Work out the finished part from the listing and answer in its coordinate system (mm). A direction names the side the tool comes from. Round coordinates to 2 decimals unless told otherwise and drop trailing zeros. Write each loop counter-clockwise with the first axis right and the second up, starting at its lowest first coordinate (ties: lowest second). Pieces come first, ordered by that corner, then holes. Notation, with made-up numbers: (-22.75, 49) -> (26.25, 49) arc R11 ccw to (26.25, 63) -> close; hole circle Ø3 at (72, -22). An arc over 180 degrees is marked (long way). Answer as a JSON object with one key per item and string values. Group by question number.
from build123d import *

# Parameters (mm, degrees)
SKETCH3_W               = 55.024039141
SKETCH3_H               = 32.210333873
BOSS_EXTRUDE1_DEPTH     = 1.5
SKETCH4_W               = 14
SKETCH4_H               = 14
CUT_EXTRUDE1_DEPTH      = 1.5
CUT_EXTRUDE4_DEPTH      = 327.051192929
CUT_EXTRUDE4_DEPTH_BACK = 327.051192929


with BuildPart() as part:
    # Sketch3 → Boss-Extrude1 (new body)
    with BuildSketch(Plane.XY):
        with Locations((282.811419242, 83.927296462)):
            Rectangle(SKETCH3_W, SKETCH3_H)
    extrude(amount=BOSS_EXTRUDE1_DEPTH)

    # Sketch4 → Cut-Extrude1 (cut)
    with BuildSketch(Plane.XY.offset(1.5)):
        with Locations((271.905830275, 82.45473243)):
            Rectangle(SKETCH4_W, SKETCH4_H)
        with Locations((290.956988381, 82.45473243)):
            Rectangle(SKETCH4_W, SKETCH4_H)
    extrude(amount=-CUT_EXTRUDE1_DEPTH, mode=Mode.SUBTRACT)

    # Sketch1 → Cut-Extrude4 (cut, two sides: drawn at the far end of the back side and taken through both)
    with BuildSketch(Plane.XY.offset(-CUT_EXTRUDE4_DEPTH_BACK)):
        Polygon((272.906316619, 84.755597823), (272.906316619, 87.985794184), (266.155906266, 87.985794184), (266.155906266, 84.755597823), (265.330856112, 84.755597823), (265.330856112, 81.955427603), (266.155906266, 81.955427603), (266.155906266, 75.684746413), (267.880011074, 75.684746413), (267.880011074, 74.484573455), (271.18021169, 74.484573455), (271.18021169, 75.684746413), (272.906316619, 75.684746413), (272.906316619, 80.155418181), (274.431409328, 80.155418181), (274.431409328, 75.45473243), (288.431409328, 75.45473243), (288.431409328, 80.155418181), (289.956502038, 80.155418181), (289.956502038, 75.684746413), (291.680606845, 75.684746413), (291.680606845, 74.484573455), (294.980807461, 74.484573455), (294.980807461, 75.684746413), (296.70691239, 75.684746413), (296.70691239, 81.955427603), (297.530962483, 81.955427603), (297.530962483, 84.755446764), (296.70691239, 84.755446764), (296.70691239, 87.985643125), (289.956502038, 87.985643125), (289.956502038, 84.755446764), (288.431409328, 84.755446764), (288.431409328, 89.45473243), (274.431409328, 89.45473243), (274.431409328, 84.755597823), align=None)
    extrude(amount=CUT_EXTRUDE4_DEPTH + CUT_EXTRUDE4_DEPTH_BACK, mode=Mode.SUBTRACT)


solid = part.part
1) A cutting plane is placed at C-C on y = 79.5. Determine the outline of the cut face in (x, z).
2) A cutting plane is placed at A-A on z = 1. Determine the outline of the cut face in (x, y), plus the area to 3 significant figures.
3) For a pull along X with two mould halves and no side action, classify faces 1 (the face through (291.681, 75, 1)), 2 (the face through (282, 67.822, 1)), 3 (the face through (310.323, 84, 1)) as released by +X, released by -X, zero draft, split by the parting line, or undercut.
4) A cutting plane is placed at B-B on x = 290. Determine the outline of the cut face in (y, z), plus the area to 3 significant figures.
5) A tool of negligible diameter and unlimited length cuts with its end or side. For faces 4 (the face through (281, 89.455, 1)), 5 (the face through (255.299, 84, 1)), from which of +Z, -Z, +X, -X, +Y, -Y can it reach the whole face along a straight path? Write none if from no direction.
6) Straight lines are drawn through the part: L1, parallel to Y at x = 287, z = 0.4; L2, parallel to X at y = 86, z = 1.1; L3, parallel to X at y = 75, z = 0.5. For each, find the intervals that lie inside material, in ascending order.
Established:
{
 "1": {"outline": "(255.3, 0) -> (264.91, 0) -> (264.91, 1.5) -> (255.3, 1.5) -> close; (297.96, 0) -> (310.32, 0) -> (310.32, 1.5) -> (297.96, 1.5) -> close"},
 "2": {"outline": "(255.3, 67.82) -> (310.32, 67.82) -> (310.32, 100.03) -> (255.3, 100.03) -> close; hole (264.91, 75.45) -> (267.88, 75.45) -> (267.88, 74.48) -> (271.18, 74.48) -> (271.18, 75.45) -> (291.68, 75.45) -> (291.68, 74.48) -> (294.98, 74.48) -> (294.98, 75.45) -> (297.96, 75.45) -> (297.96, 89.45) -> (264.91, 89.45) -> close", "area": "1,300 mm²"},
 "3": {"face 1": "undercut", "face 2": "zero draft", "face 3": "released by +X"},
 "4": {"outline": "(67.82, 0) -> (75.45, 0) -> (75.45, 1.5) -> (67.82, 1.5) -> close; (89.45, 0) -> (100.03, 0) -> (100.03, 1.5) -> (89.45, 1.5) -> close", "area": "27.3 mm²"},
 "5": {"face 4": "+Z, -Z", "face 5": "+Z, -Z, -X, +Y, -Y"},
 "6": {"L1": "y = 67.82 to 75.45, 89.45 to 100.03", "L2": "x = 255.3 to 264.91, 297.96 to 310.32", "L3": "x = 255.3 to 267.88, 271.18 to 291.68, 294.98 to 310.32"}
}
